Check sheet for the drawn part. Datum: minimum x, y, z corner. Units: mm. A direction names the side the tool comes from. Round coordinates to 2 decimals unless told otherwise and drop trailing zeros. Write each loop counter-clockwise with the first axis right and the second up, starting at its lowest first coordinate (ties: lowest second). Pieces come first, ordered by that corner, then holes.
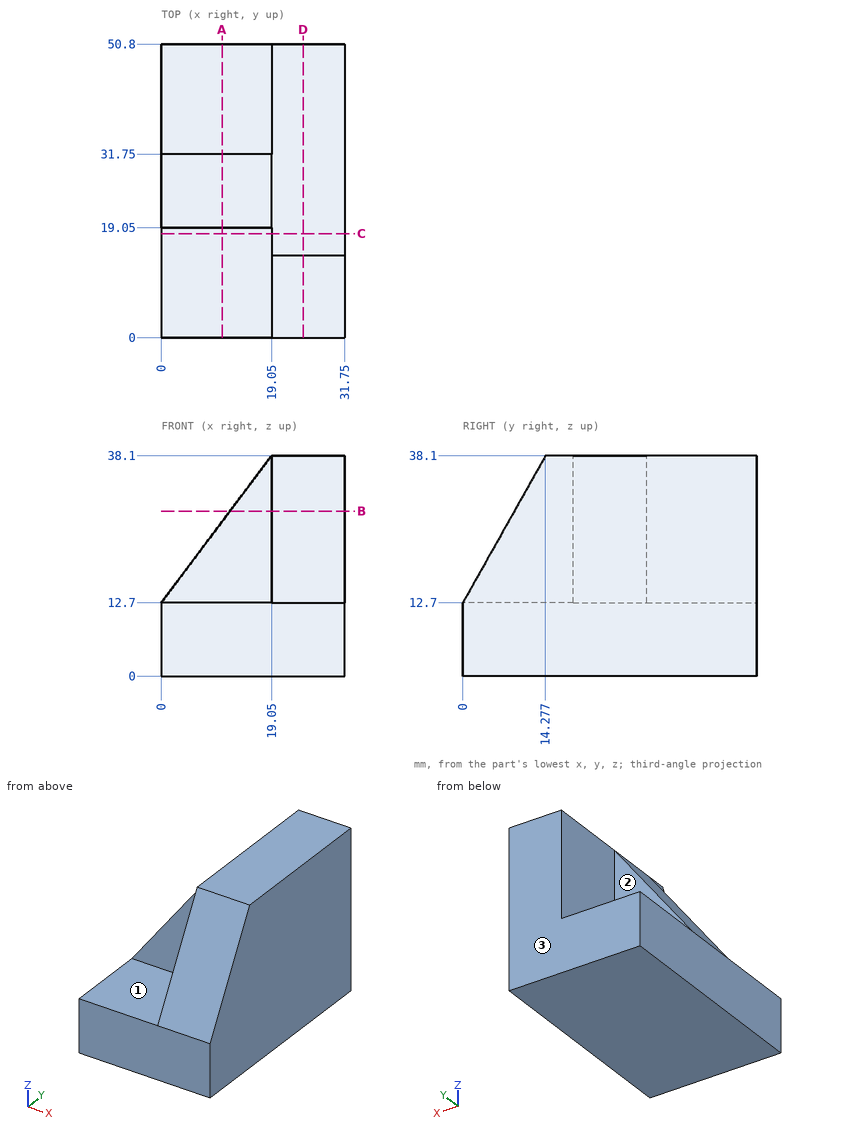
Q1. Sectioned sample at D-D (x = 24.5). Enter the section's corners in (y, z).
Recorded:
outline: (0, 0) - (50.8, 0) - (50.8, 38.1) - (14.28, 38.1) - (0, 12.7) - close
Q2. Material ranges on line 1 along Z through (x, y) = (5, 42); line 2 along Y through (x, z) = (11, 13), recorded low to high.
Recorded:
line 1: z = 0 to 12.7
line 2: y = 19.05 to 31.75
Q3. Sectioned sample at C-C (y = 18). Enter the section's corners in (x, z).
Recorded:
outline: (0, 0) - (31.75, 0) - (31.75, 38.1) - (19.05, 38.1) - (19.05, 12.7) - (0, 12.7) - close
Q4. Depth check by flat-ended pin: P1, Ø5.5, axis at x = 6, z = 22.5, coming from the +Y side; P2, Ø1, axis at x = 13.5, y = 26, coming from the +Z side (1 decimal); P3, Ø3, axis at x = 8.5, y = 26.5, coming from the +Z side (1 decimal); P4, Ø12, axis at x = 22, z = 4.5, coming from the -Y side. Enter the tip coordinate at first touch or a pass-through.
Recorded:
P1: stops at y = 31.75
P2: stops at z = 31.4
P3: stops at z = 26
P4: stops at y = 0
Q5. Sectioned sample at B-B (z = 28.5). Enter the section's corners in (x, y).
Recorded:
outline: (11.85, 19.05) - (19.05, 19.05) - (19.05, 8.88) - (31.75, 8.88) - (31.75, 50.8) - (19.05, 50.8) - (19.05, 31.75) - (11.85, 31.75) - close
Q6. Tool access check on the marked faces 1, 2 and 3. Record the directions out of +Z, -Z, +X, -X, +Y, -Y that give a thin tool (end or side, any length) a straight path to the whole face; none if there is none.
Recorded:
face 1: +Z, -X, -Y
face 2: +Z, -X, +Y
face 3: +Z, -Z, +X, -X, +Y
Q7. Sectioned sample at A-A (x = 10.5). Enter the section's corners in (y, z), plus the area to 3 significant figures.
Recorded:
outline: (0, 0) - (50.8, 0) - (50.8, 12.7) - (31.75, 12.7) - (31.75, 26.7) - (19.05, 26.7) - (19.05, 12.7) - (0, 12.7) - close
area: 823 mm2
